Check sheet for the modelled part. Datum: model origin and axes. Units: mm. A direction names the side the tool comes from. Coordinates: 2 decimals unless noted, no trailing zeros. Loops run counter-clockwise (first coordinate to the right, second up) from the corner with the lowest first, then second, coordinate; pieces in that order, holes last. Notation, with made-up numbers: (23, 24.25) -> (46, 24.25) arc R26 cw to (46, 61.25) -> close; hole circle Ø5 at (-23.75, 76). An arc over 180 degrees is marked (long way). Use CSV: the item, a comma, the result in double quotes.
```python
from build123d import *

# Parameters (mm, degrees)
ESBO_O1_W                        = 47.5
ESBO_O1_H                        = 39
FLANGE_BASE1_DEPTH               = 3
ESBO_O6_R                        = 2.3
CORTE_EXTRUS_O1_DEPTH            = 10
ARESTA_FLANGE1_STRIP_W           = 13.4732
ARESTA_FLANGE1_STRIP_H           = 3
ARESTA_FLANGE1_STRIP_CUT_DEPTH   = 39
ARESTA_FLANGE1_STRIP_2_W         = 13.4732
ARESTA_FLANGE1_STRIP_2_H         = 3
ARESTA_FLANGE1_STRIP_CUT_2_DEPTH = 39
ARESTA_FLANGE1_DEPTH             = 39
ARESTA_FLANGE1_BEND_DEPTH        = 39
ESBO_O13_R                       = 2
ESBO_O13_R_2                     = 0.75
CORTE_EXTRUS_O2_DEPTH            = 70
FILETE1_R                        = 5
ESBO_O14_R                       = 1.997873176
ESBO_O14_R_2                     = 2.026064888
ESBO_O14_R_3                     = 2
CORTE_EXTRUS_O4_DEPTH            = 3
BOSS_EXTRUDE1_START              = 0.5
SKETCH1_R                        = 2.5
SKETCH1_R_2                      = 2
BOSS_EXTRUDE1_DEPTH              = 0.5
SKETCH2_R                        = 4
CUT_EXTRUDE8_DEPTH               = 2
CORTE_EXTRUS_O5_REACH            = 66.966
ESBO_O15_R                       = 2


# Sheet-metal steps are written as plain solids
with BuildPart() as part:
    # Esboço1 → Flange-base1 (new body)
    with BuildSketch(Plane.XY):
        with Locations((3.243735783, -4.490936556)):
            Rectangle(ESBO_O1_W, ESBO_O1_H)
    extrude(amount=-FLANGE_BASE1_DEPTH)

    # Esboço6 → Corte-extrusão1 (cut)
    with BuildSketch(Plane.XY):
        with BuildLine():
            Line((-13.656264217, 10.009063444), (-13.656264217, 12.009063444))
            Line((-13.656264217, 12.009063444), (-11.656264217, 12.009063444))
            ThreePointArc((-11.656264217, 12.009063444), (-15.070477779, 13.423277006), (-13.656264217, 10.009063444))
        make_face()
        with BuildLine():
            Line((-11.656264217, 12.009063444), (-13.656264217, 12.009063444))
            Line((-13.656264217, 12.009063444), (-13.656264217, 10.009063444))
            ThreePointArc((-13.656264217, 10.009063444), (-12.242050654, 10.594849882), (-11.656264217, 12.009063444))
        make_face()
        with BuildLine():
            ThreePointArc((-11.656264217, -16.490936556), (-12.242050654, -15.076722994), (-13.656264217, -14.490936556))
            Line((-13.656264217, -14.490936556), (-13.656264217, -16.490936556))
            Line((-13.656264217, -16.490936556), (-11.656264217, -16.490936556))
        make_face()
        with BuildLine():
            Line((-13.656264217, -16.490936556), (-13.656264217, -14.490936556))
            ThreePointArc((-13.656264217, -14.490936556), (-15.070477779, -17.905150118), (-11.656264217, -16.490936556))
            Line((-11.656264217, -16.490936556), (-13.656264217, -16.490936556))
        make_face()
        with Locations((3.243735783, -4.490936556)):
            Circle(ESBO_O6_R)
        with BuildLine():
            Line((4.993735783, 12.009063444), (1.493735783, 12.009063444))
            Line((1.493735783, 12.009063444), (1.493735783, 3.523823043))
            ThreePointArc((1.493735783, 3.523823043), (3.243735783, 1.773823043), (4.993735783, 3.523823043))
            Line((4.993735783, 3.523823043), (4.993735783, 12.009063444))
        make_face()
        with BuildLine():
            Line((1.493735783, 12.523823043), (1.493735783, 12.009063444))
            Line((1.493735783, 12.009063444), (4.993735783, 12.009063444))
            Line((4.993735783, 12.009063444), (4.993735783, 12.523823043))
            ThreePointArc((4.993735783, 12.523823043), (3.243735783, 14.273823043), (1.493735783, 12.523823043))
        make_face()
        with BuildLine():
            Line((1.493735783, -12.505696155), (1.493735783, -16.490936556))
            Line((1.493735783, -16.490936556), (4.993735783, -16.490936556))
            Line((4.993735783, -16.490936556), (4.993735783, -12.505696155))
            ThreePointArc((4.993735783, -12.505696155), (3.243735783, -10.755696155), (1.493735783, -12.505696155))
        make_face()
        with BuildLine():
            Line((4.993735783, -16.490936556), (1.493735783, -16.490936556))
            Line((1.493735783, -16.490936556), (1.493735783, -21.505696155))
            ThreePointArc((1.493735783, -21.505696155), (3.243735783, -23.255696155), (4.993735783, -21.505696155))
            Line((4.993735783, -21.505696155), (4.993735783, -16.490936556))
        make_face()
        with BuildLine():
            ThreePointArc((22.143735783, -16.490936556), (21.557949346, -15.076722994), (20.143735783, -14.490936556))
            Line((20.143735783, -14.490936556), (20.143735783, -16.490936556))
            Line((20.143735783, -16.490936556), (18.143735783, -16.490936556))
            ThreePointArc((18.143735783, -16.490936556), (20.143735783, -18.490936556), (22.143735783, -16.490936556))
        make_face()
        with BuildLine():
            Line((20.143735783, -16.490936556), (20.143735783, -14.490936556))
            ThreePointArc((20.143735783, -14.490936556), (18.729522221, -15.076722994), (18.143735783, -16.490936556))
            Line((18.143735783, -16.490936556), (20.143735783, -16.490936556))
        make_face()
        with BuildLine():
            ThreePointArc((22.143735783, 12.009063444), (20.143735783, 14.009063444), (18.143735783, 12.009063444))
            Line((18.143735783, 12.009063444), (20.143735783, 12.009063444))
            Line((20.143735783, 12.009063444), (20.143735783, 10.009063444))
            ThreePointArc((20.143735783, 10.009063444), (21.557949346, 10.594849882), (22.143735783, 12.009063444))
        make_face()
        with BuildLine():
            Line((20.143735783, 12.009063444), (18.143735783, 12.009063444))
            ThreePointArc((18.143735783, 12.009063444), (18.729522221, 10.594849882), (20.143735783, 10.009063444))
            Line((20.143735783, 10.009063444), (20.143735783, 12.009063444))
        make_face()
    extrude(amount=-CORTE_EXTRUS_O1_DEPTH, mode=Mode.SUBTRACT)

    # Aresta-Flange1 strip (across the edge) → Aresta-Flange1 strip cut (cut)
    with BuildSketch(Plane(origin=(26.993735783, -23.990936556, 0), x_dir=(-1, 0, 0), z_dir=(0, 1, 0))):
        with Locations((-6, -1.5)):
            Rectangle(ARESTA_FLANGE1_STRIP_W, ARESTA_FLANGE1_STRIP_H)
    extrude(amount=ARESTA_FLANGE1_STRIP_CUT_DEPTH, mode=Mode.SUBTRACT)

    # Aresta-Flange1 strip 2 (across the edge) → Aresta-Flange1 strip cut 2 (cut)
    with BuildSketch(Plane(origin=(-20.506264217, 15.009063444, 0), x_dir=(1, 0, 0), z_dir=(0, -1, 0))):
        with Locations((-6, -1.5)):
            Rectangle(ARESTA_FLANGE1_STRIP_2_W, ARESTA_FLANGE1_STRIP_2_H)
    extrude(amount=ARESTA_FLANGE1_STRIP_CUT_2_DEPTH, mode=Mode.SUBTRACT)

    # Aresta-Flange1 section (across the edge) → Aresta-Flange1 (add)
    with BuildSketch(Plane(origin=(26.993735783, -23.990936556, 0), x_dir=(-1, 0, 0), z_dir=(0, 1, 0))):
        with BuildLine():
            Line((-3, 0.7366), (-3, 27))
            Line((-3, 27), (0, 27))
            Line((0, 27), (0, 0.7366))
            ThreePointArc((0, 0.7366), (0.215745145, 0.215745145), (0.7366, 0))
            Line((0.7366, 0), (0.7366, -3))
            ThreePointArc((0.7366, -3), (-1.905575199, -1.905575199), (-3, 0.7366))
        make_face()
    extrude(amount=ARESTA_FLANGE1_DEPTH)

    # Aresta-Flange1 section 2 (across the edge) → Aresta-Flange1 bend (add)
    with BuildSketch(Plane(origin=(-20.506264217, 15.009063444, 0), x_dir=(1, 0, 0), z_dir=(0, -1, 0))):
        with BuildLine():
            Line((-3, 0.7366), (-3, 27))
            Line((-3, 27), (0, 27))
            Line((0, 27), (0, 0.7366))
            ThreePointArc((0, 0.7366), (0.215745145, 0.215745145), (0.7366, 0))
            Line((0.7366, 0), (0.7366, -3))
            ThreePointArc((0.7366, -3), (-1.905575199, -1.905575199), (-3, 0.7366))
        make_face()
    extrude(amount=ARESTA_FLANGE1_BEND_DEPTH)

    # Esboço13 → Corte-extrusão2 (cut)
    with BuildSketch(Plane.ZY.offset(23.506264217)):
        with Locations((21.734737, -7.820936556)):
            Circle(ESBO_O13_R)
        with Locations((21.734737, 0.629063444)):
            Circle(ESBO_O13_R_2)
        Polygon((0.7366, -23.990936556), (27, -23.990936556), (27, -10.990936556), align=None)
    extrude(amount=-CORTE_EXTRUS_O2_DEPTH, mode=Mode.SUBTRACT)

    # Filete1
    filete1_edges = [part.edges().sort_by_distance(p)[0] for p in [
        (28.493735783, 15.009063444, 27),
        (-22.006264217, 15.009063444, 27),
        (-22.006264217, -10.990936556, 27),
        (28.493735783, -10.990936556, 27),
    ]]
    fillet(filete1_edges, radius=FILETE1_R)

    # Esboço14 → Corte-extrusão4 (cut)
    with BuildSketch(Plane.XY):
        with Locations((-5.331264217, 12.009063444)):
            Circle(ESBO_O14_R)
        with Locations((11.818735783, 12.009063444)):
            Circle(ESBO_O14_R_2)
        with Locations((13.743735783, -2.990936556)):
            Circle(ESBO_O14_R_3)
        with Locations(Location((-7.256264217, -2.990936556, 0), (0, 0, 180))):
            Circle(ESBO_O14_R_3)
    extrude(amount=-CORTE_EXTRUS_O4_DEPTH, mode=Mode.SUBTRACT)

    # Sketch1 → Boss-Extrude1 (add)
    with BuildSketch(Plane.ZY.offset(23.506264217).offset(BOSS_EXTRUDE1_START)):
        with Locations(Location((21.734737, -7.820936556, 0), (0, 0, 180))):
            Circle(SKETCH1_R)
        with Locations((21.734737, -7.820936556)):
            Circle(SKETCH1_R_2, mode=Mode.SUBTRACT)
    boss_extrude1 = extrude(amount=-BOSS_EXTRUDE1_DEPTH)

    # Sketch2 → Cut-Extrude8 (cut)
    with BuildSketch(Plane(origin=(-20.506264217, 0, 0), x_dir=(0, 0, -1), z_dir=(1, 0, 0))):
        with Locations((-21.734737, -7.820936556)):
            Circle(SKETCH2_R)
    cut_extrude8 = extrude(amount=-CUT_EXTRUDE8_DEPTH, mode=Mode.SUBTRACT)

    # Mirror1: Boss-Extrude1, Cut-Extrude8 across plane
    add(boss_extrude1.mirror(Plane.ZY.offset(-3.243735783)))
    add(cut_extrude8.mirror(Plane.ZY.offset(-3.243735783)), mode=Mode.SUBTRACT)

    # Corte-extrusão5: up to this face of the body (flat: up to its plane)
    corte_extrus_o5_end = Plane(part.part.faces().sort_by_distance((-23.506264217, -1.392336246, 12.655784695))[0])
    # Esboço15 → Corte-extrusão5 (cut, up to the picked face)
    with BuildSketch(Plane(origin=(29.993735783, 0, 0), x_dir=(0, 0, -1), z_dir=(1, 0, 0)), mode=Mode.PRIVATE) as corte_extrus_o5_sk1:
        with Locations((-4.2366, -3.490936556)):
            Circle(ESBO_O15_R)
    corte_extrus_o5_tool1 = split(extrude(corte_extrus_o5_sk1.sketch, amount=-CORTE_EXTRUS_O5_REACH, mode=Mode.PRIVATE), bisect_by=corte_extrus_o5_end, keep=Keep.BOTH, mode=Mode.PRIVATE)
    add(corte_extrus_o5_tool1.solids().sort_by(Axis((29.993736, -3.490937, 4.2366), (-1, 0, 0)))[0], mode=Mode.SUBTRACT)


solid = part.part
```
1) Go/stop test with flat-tipped pins: pin 1 Ø1 at (y, z) = (-3.5, 11.5) entering from -X; pin 2 Ø5 at (x, y) = (-13.66, -16.49) entering from +Z; pin 3 Ø1 at (y, z) = (-11, 2.5) entering from +X. Record where each tip stops, or that it passes through.
Answer below:
pin 1,"stops at x = -23.51"
pin 2,"stops at z = 0"
pin 3,"stops at x = 29.99"
2) Cross-section at B-B on z = 5.5. Record the boundary of the cut face in (x, y), and give its area (3 significant figures).
Answer below:
outline,"(-23.51, -21.63) -> (-20.51, -21.63) -> (-20.51, -5.04) -> (-23.51, -5.04) -> close; (-23.51, -1.94) -> (-20.51, -1.94) -> (-20.51, 15.01) -> (-23.51, 15.01) -> close; (26.99, -21.63) -> (29.99, -21.63) -> (29.99, -5.04) -> (26.99, -5.04) -> close; (26.99, -1.94) -> (29.99, -1.94) -> (29.99, 15.01) -> (26.99, 15.01) -> close"
area,"201 mm²"
3) Cross-section at D-D on y = -17.5. Record the boundary of the cut face in (x, z).
Answer below:
outline,"(-23.51, 0.74) arc R3.74 ccw to (-19.77, -3) -> (-15.38, -3) -> (-15.38, 0) -> (-19.77, 0) arc R0.74 cw to (-20.51, 0.74) -> (-20.51, 13.85) -> (-23.51, 13.85) -> close; (-11.93, -3) -> (1.49, -3) -> (1.49, 0) -> (-11.93, 0) -> close; (4.99, -3) -> (18.42, -3) -> (18.42, 0) -> (4.99, 0) -> close; (21.87, -3) -> (26.26, -3) arc R3.74 ccw to (29.99, 0.74) -> (29.99, 13.85) -> (26.99, 13.85) -> (26.99, 0.74) arc R0.74 cw to (26.26, 0) -> (21.87, 0) -> close"
4) Access from +Z, -Z, +X, -X, +Y, -Y to the whole of each face (thin tool, end or side, straight path). Record for faces 1 (the cylindrical face through (-23.76, -7.931, 24.232)), 2 (the cylindrical face through (3.282, 14.273, -1.479)), 3 (the flat face through (28.994, -9, 24)), 4 (the cylindrical face through (30.247, -7.931, 24.232)), 5 (the flat face through (26.994, 0, 14)).
Answer below:
face 1,"-X"
face 2,"+Z, -Z"
face 3,"none"
face 4,"+X"
face 5,"+Z, +Y, -Y"
5) Cross-section at A-A on y = 8.5. Record the boundary of the cut face in (x, z).
Answer below:
outline,"(-23.51, 0.74) arc R3.74 ccw to (-19.77, -3) -> (1.49, -3) -> (1.49, 0) -> (-19.77, 0) arc R0.74 cw to (-20.51, 0.74) -> (-20.51, 27) -> (-23.51, 27) -> close; (4.99, -3) -> (26.26, -3) arc R3.74 ccw to (29.99, 0.74) -> (29.99, 27) -> (26.99, 27) -> (26.99, 0.74) arc R0.74 cw to (26.26, 0) -> (4.99, 0) -> close"
6) Thickness scan on line 1 along X through (y, z) = (11, 15.75); line 2 along X through (y, z) = (-9, 25.5); line 3 along Z through (x, y) = (18.5, -2). Record the ranges inside material, lowest first. Write a range as from..to.
Answer below:
line 1,"x = -23.51..-20.51, 26.99..29.99"
line 2,"x = -23.51..-22.51, 28.99..29.99"
line 3,"z = -3..0"
7) Cross-section at C-C on x = 21. Record the boundary of the cut face in (y, z).
Answer below:
outline,"(-23.99, -3) -> (-18.3, -3) -> (-18.3, 0) -> (-23.99, 0) -> close; (-14.68, -3) -> (10.2, -3) -> (10.2, 0) -> (-14.68, 0) -> close; (13.82, -3) -> (15.01, -3) -> (15.01, 0) -> (13.82, 0) -> close"
8) Draft check along Z on faces 6 (the cylindrical face through (-21.99, 13.58, 25.5)), 7 (the cylindrical face through (-23.267, -7.733, 19.737)), 8 (the flat face through (-20.506, 0, 14)). Enter one of: released by +Z, released by -Z, zero draft, split by the parting line, or undercut.
Answer below:
face 6,"released by +Z"
face 7,"undercut"
face 8,"zero draft"
